Design review of the part built by this model. Coordinates are the model's own, in mm. Coordinates: 2 decimals unless noted, no trailing zeros. Write each loop counter-clockwise with the first axis right and the second up, starting at its lowest first coordinate (ties: lowest second). Pieces come first, ordered by that corner, then holes.
Q1. For L1, parallel to X at y = -3.5, z = -33; L2, parallel to X at y = -0.75, z = -99; L3, parallel to X at y = -4.5, z = -22, list the stretches that pass through material, from the lowest coordinate up.
Q2. Take a section at B-B, the plane x = 9.5. Write out the cut boundary in (y, z) (3 decimals), plus the area to 3 significant figures.
Q3. For pin 1 Ø0.8 at (x, y) = (30.5, -4.5) entering from +Z (3 decimals), flat-tipped, find the tip position at first contact; note if it passes through.
from build123d import *

# Parameters (mm, degrees)
SKETCH1_W      = 76.454
SKETCH1_H      = 106.3752
EXTRUDE1_DEPTH = 6.223
SKETCH2_W      = 6.35
SKETCH2_H      = 14.732
EXTRUDE2_DEPTH = 132.147333256
SKETCH3_R      = 0.8128
EXTRUDE3_DEPTH = 9.525
SKETCH5_R      = 0.8128
EXTRUDE4_DEPTH = 132.147333256
SKETCH7_W      = 63.754
SKETCH7_H      = 0.79375
EXTRUDE5_DEPTH = 0.79375
CHAMFER1_SIZE  = 0.1778
SKETCH8_W      = 6.35
SKETCH8_H      = 106.3752
EXTRUDE7_DEPTH = 1.905


with BuildPart() as part:
    # Sketch1 → Extrude1 (new body)
    with BuildSketch(Plane(origin=(0, 0, 0), x_dir=(1, 0, 0), z_dir=(0, 1, 0))):
        with Locations((38.227, 53.1876)):
            Rectangle(SKETCH1_W, SKETCH1_H)
    extrude(amount=-EXTRUDE1_DEPTH)

    # Sketch2 → Extrude2 (cut, through all)
    with BuildSketch(Plane(origin=(0, 0, 0), x_dir=(-1, 0, 0), z_dir=(0, 1, 0))):
        with Locations((-3.175, -7.366)):
            Rectangle(SKETCH2_W, SKETCH2_H)
        with Locations((-73.279, -7.366)):
            Rectangle(SKETCH2_W, SKETCH2_H)
        with Locations((-73.279, -99.0092)):
            Rectangle(SKETCH2_W, SKETCH2_H)
        with Locations((-3.175, -99.0092)):
            Rectangle(SKETCH2_W, SKETCH2_H)
    extrude(amount=-EXTRUDE2_DEPTH, mode=Mode.SUBTRACT)

    # Sketch3 → Extrude3 (cut)
    with BuildSketch(Plane.XY):
        with Locations((15.367, -4.6355)):
            Circle(SKETCH3_R)
        with Locations((22.987, -4.6355)):
            Circle(SKETCH3_R)
        with Locations((30.607, -4.6355)):
            Circle(SKETCH3_R)
        with Locations((38.227, -4.6355)):
            Circle(SKETCH3_R)
        with Locations((45.847, -4.6355)):
            Circle(SKETCH3_R)
        with Locations((53.467, -4.6355)):
            Circle(SKETCH3_R)
        with Locations((61.087, -4.6355)):
            Circle(SKETCH3_R)
    extrude(amount=-EXTRUDE3_DEPTH, mode=Mode.SUBTRACT)

    # Sketch5 → Extrude4 (cut, through all)
    with BuildSketch(Plane(origin=(0, 0, 0), x_dir=(1, 0, 0), z_dir=(0, 1, 0))):
        with Locations(Location((1.28905, 83.6676, 0), (0, 0, 270))):
            Circle(SKETCH5_R)
        with Locations(Location((1.28905, 63.3476, 0), (0, 0, 270))):
            Circle(SKETCH5_R)
        with Locations(Location((1.28905, 53.1876, 0), (0, 0, 270))):
            Circle(SKETCH5_R)
        with Locations(Location((1.28905, 73.5076, 0), (0, 0, 270))):
            Circle(SKETCH5_R)
        with Locations(Location((1.28905, 32.8676, 0), (0, 0, 270))):
            Circle(SKETCH5_R)
        with Locations(Location((1.28905, 22.7076, 0), (0, 0, 270))):
            Circle(SKETCH5_R)
        with Locations(Location((75.16495, 83.6676, 0), (0, 0, 90))):
            Circle(SKETCH5_R)
        with Locations(Location((75.16495, 73.5076, 0), (0, 0, 90))):
            Circle(SKETCH5_R)
        with Locations(Location((75.16495, 63.3476, 0), (0, 0, 90))):
            Circle(SKETCH5_R)
        with Locations(Location((75.16495, 53.1876, 0), (0, 0, 90))):
            Circle(SKETCH5_R)
        with Locations(Location((75.16495, 43.0276, 0), (0, 0, 90))):
            Circle(SKETCH5_R)
        with Locations(Location((75.16495, 32.8676, 0), (0, 0, 90))):
            Circle(SKETCH5_R)
        with Locations(Location((75.16495, 22.7076, 0), (0, 0, 90))):
            Circle(SKETCH5_R)
        with Locations(Location((1.28905, 43.0276, 0), (0, 0, 270))):
            Circle(SKETCH5_R)
    extrude(amount=-EXTRUDE4_DEPTH, mode=Mode.SUBTRACT)

    # Sketch7 → Extrude5 (cut)
    with BuildSketch(Plane.XZ.offset(6.223)):
        with Locations((38.227, -105.5878)):
            Rectangle(SKETCH7_W, SKETCH7_H)
    extrude(amount=-EXTRUDE5_DEPTH, mode=Mode.SUBTRACT)

    # Chamfer1
    chamfer1_edges = [part.edges().sort_by_distance(p)[0] for p in [
        (38.227, -5.42925, -105.190925),
        (38.227, -5.42925, -105.984675),
        (38.227, -6.223, -105.984675),
        (38.227, -6.223, -105.190925),
    ]]
    chamfer(chamfer1_edges, length=CHAMFER1_SIZE)

    # Sketch8 → Extrude7 (cut)
    with BuildSketch(Plane(origin=(0, 0, 0), x_dir=(-1, 0, 0), z_dir=(0, 1, 0))):
        Polygon((-10.922, 0), (-10.922, -106.3752), (-6.35, -106.3752), (-6.35, -91.6432), (-4.572, -91.6432), (-4.572, -14.732), (-6.35, -14.732), (-6.35, 0), align=None)
        with Locations((-17.907, -53.1876)):
            Rectangle(SKETCH8_W, SKETCH8_H)
        with Locations((-28.067, -53.1876)):
            Rectangle(SKETCH8_W, SKETCH8_H)
        with Locations((-38.227, -53.1876)):
            Rectangle(SKETCH8_W, SKETCH8_H)
        with Locations((-58.547, -53.1876)):
            Rectangle(SKETCH8_W, SKETCH8_H)
        Polygon((-70.104, -106.3752), (-65.532, -106.3752), (-65.532, 0), (-70.104, 0), (-70.104, -14.732), (-71.882, -14.732), (-71.882, -91.6432), (-70.104, -91.6432), align=None)
        with Locations((-48.387, -53.1876)):
            Rectangle(SKETCH8_W, SKETCH8_H)
    extrude(amount=-EXTRUDE7_DEPTH, mode=Mode.SUBTRACT)


solid = part.part
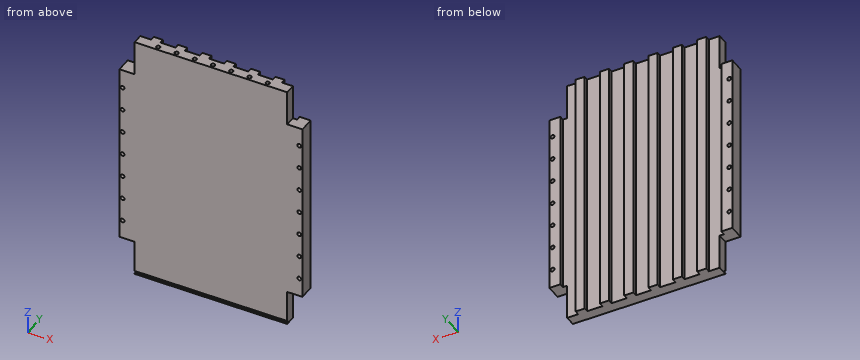
Responses:
1. L1: x = 0 to 0.49, 2.09 to 74.36, 75.97 to 76.45
1. L2: x = 10.92 to 14.73, 21.08 to 24.89, 31.24 to 35.05, 41.4 to 45.21, 51.56 to 55.37, 61.72 to 65.53
1. L3: x = 0 to 0.89, 1.69 to 74.77, 75.56 to 76.45
2. outline: (-6.223, -106.375) - (-1.905, -106.375) - (-1.905, 0) - (-6.223, 0) - (-6.223, -105.013) - (-6.045, -105.191) - (-5.607, -105.191) - (-5.429, -105.369) - (-5.429, -105.807) - (-5.607, -105.985) - (-6.045, -105.985) - (-6.223, -106.162) - close
2. area: 459 mm2
3. pin 1: stops at z = -9.525
